Work out the finished part from the listing and answer in its coordinate system (mm). A direction names the side the tool comes from. Round coordinates to 2 decimals unless told otherwise and drop trailing zeros. Write each loop counter-clockwise with the first axis right and the second up, starting at its lowest first coordinate (ties: lowest second). Pieces come first, ordered by that corner, then holes.
1. A tool of negligible diameter and unlimited length cuts with its end or side. For faces 5 (the face through (-43.452, 82.23, 13.548)), 6 (the face through (-59, 67, 0)), from which of +Z, -Z, +X, -X, +Y, -Y can it reach the whole face along a straight path? Write none if from no direction.
2. Straight lines are drawn through the part: probe 1 along X at (y, z) = (85.5, 13.75); probe 2 along X at (y, z) = (78, 7.75); probe 3 along Y at (x, z) = (-16, 16.25). For each, find the intervals that lie inside material, in ascending order.
3. Flat-ended cylindrical pins translate along their axes: pin 1 Ø8.5 at (x, z) = (-47.32, 10) entering from +Y; pin 2 Ø6.5 at (x, z) = (-16.5, 10) entering from +Y. Find the tip coordinate at first contact, or state that the pin passes through.
4. Find section A-A (z = 10). Write down the section's boundary in (x, y), and give its area (3 significant figures).
5. Determine the mould class of faces 1 (the face through (-14, 76.59, 10)), 2 (the face through (-55, 92.09, 10)), 3 (the face through (69.336, 67, 10)), 4 (the face through (-182.821, 67, 10)) for opening direction X: pulls with the +X half, pulls with the -X half, needs draft (parallel to the pull), parting line crosses it, or undercut.
```python
from build123d import *

# Parameters (mm, degrees)
BOSS_EXTRUDE1_DEPTH = 20
SKETCH5_R           = 5.25
CUT_EXTRUDE4_DEPTH  = 20
SKETCH6_W           = 13
SKETCH6_H           = 13
CUT_EXTRUDE5_DEPTH  = 15.5
SKETCH7_W           = 13
SKETCH7_H           = 13
CUT_EXTRUDE6_DEPTH  = 15.5
SKETCH8_W           = 300
SKETCH8_H           = 102
BOSS_EXTRUDE2_DEPTH = 20
CUT_EXTRUDE7_START  = -150
SKETCH9_W           = 47.842391085
SKETCH9_H           = 20
CUT_EXTRUDE7_DEPTH  = 150
SKETCH10_W          = 252.157608915
SKETCH10_H          = 50
CUT_EXTRUDE8_DEPTH  = 310
SKETCH11_W          = 252.157608915
SKETCH11_H          = 50
CUT_EXTRUDE9_DEPTH  = 20


with BuildPart() as part:
    # Sketch1 → Boss-Extrude1 (new body)
    with BuildSketch(Plane.XY):
        Polygon((-107.821386225, 92.09039548), (-7.821386225, 92.09039548), (117.178613775, 92.09039548), (117.178613775, 44.09039548), (-7.821386225, 44.09039548), (-107.821386225, 44.09039548), (-182.821386225, 44.09039548), (-182.821386225, 92.09039548), align=None)
    extrude(amount=BOSS_EXTRUDE1_DEPTH)

    # Sketch5 → Cut-Extrude4 (cut)
    with BuildSketch(Plane(origin=(0, 92.09039548, 0), x_dir=(1, 0, 0), z_dir=(0, 1, 0))):
        with Locations(Location((-66.321386225, -10, 0), (0, 0, 180))):
            Circle(SKETCH5_R)
        with Locations(Location((-47.321386225, -10, 0), (0, 0, 180))):
            Circle(SKETCH5_R)
    extrude(amount=-CUT_EXTRUDE4_DEPTH, mode=Mode.SUBTRACT)

    # Sketch6 → Cut-Extrude5 (cut)
    with BuildSketch(Plane(origin=(0, 92.09039548, 0), x_dir=(1, 0, 0), z_dir=(0, 1, 0))):
        with Locations((-99.441386225, -10.25)):
            Rectangle(SKETCH6_W, SKETCH6_H)
    extrude(amount=-CUT_EXTRUDE5_DEPTH, mode=Mode.SUBTRACT)

    # Sketch7 → Cut-Extrude6 (cut)
    with BuildSketch(Plane(origin=(0, 92.09039548, 0), x_dir=(1, 0, 0), z_dir=(0, 1, 0))):
        with Locations((-14.16377731, -10.25)):
            Rectangle(SKETCH7_W, SKETCH7_H)
    extrude(amount=-CUT_EXTRUDE6_DEPTH, mode=Mode.SUBTRACT)

    # Sketch8 → Boss-Extrude2 (add)
    with BuildSketch(Plane.XY.offset(20)):
        with Locations((-32.821386225, -6.90960452)):
            Rectangle(SKETCH8_W, SKETCH8_H)
    extrude(amount=-BOSS_EXTRUDE2_DEPTH)

    # Sketch9 → Cut-Extrude7 (cut)
    with BuildSketch(Plane(origin=(0, 92.09039548, 0), x_dir=(1, 0, 0), z_dir=(0, 1, 0)).offset(CUT_EXTRUDE7_START)):
        with Locations((93.257418233, -10)):
            Rectangle(SKETCH9_W, SKETCH9_H)
    extrude(amount=CUT_EXTRUDE7_DEPTH, mode=Mode.SUBTRACT)

    # Sketch10 → Cut-Extrude8 (cut)
    with BuildSketch(Plane(origin=(0, 0, 0), x_dir=(-1, 0, 0), z_dir=(0, 0, -1))):
        with Locations((56.742581767, -32.90960452)):
            Rectangle(SKETCH10_W, SKETCH10_H)
    extrude(amount=-CUT_EXTRUDE8_DEPTH, mode=Mode.SUBTRACT)

    # Sketch11 → Cut-Extrude9 (cut)
    with BuildSketch(Plane(origin=(0, 0, 0), x_dir=(-1, 0, 0), z_dir=(0, 0, -1))):
        with Locations((56.742581767, 17.09039548)):
            Rectangle(SKETCH11_W, SKETCH11_H)
    extrude(amount=-CUT_EXTRUDE9_DEPTH, mode=Mode.SUBTRACT)


solid = part.part
```
Worked answers:
1. face 5: +Y
1. face 6: -Z, +X, -X, +Y, -Y
2. probe 1: x = -182.82 to -105.94, -92.94 to -70, -62.65 to -51, -43.65 to -20.66, -7.66 to 69.34
2. probe 2: x = -182.82 to -105.94, -92.94 to -71.06, -61.58 to -52.06, -42.58 to -20.66, -7.66 to 69.34
2. probe 3: y = 42.09 to 76.59
3. pin 1: stops at y = 72.09
3. pin 2: stops at y = 76.59
4. outline: (-182.82, 42.09) - (69.34, 42.09) - (69.34, 92.09) - (-7.66, 92.09) - (-7.66, 76.59) - (-20.66, 76.59) - (-20.66, 92.09) - (-42.07, 92.09) - (-42.07, 72.09) - (-52.57, 72.09) - (-52.57, 92.09) - (-61.07, 92.09) - (-61.07, 72.09) - (-71.57, 72.09) - (-71.57, 92.09) - (-92.94, 92.09) - (-92.94, 76.59) - (-105.94, 76.59) - (-105.94, 92.09) - (-182.82, 92.09) - close
4. area: 11,800 mm2
5. face 1: undercut
5. face 2: needs draft
5. face 3: pulls with the +X half
5. face 4: pulls with the -X half
